from build123d import *

# Parameters (mm, degrees)
BOSS_EXTRUDE1_DEPTH      = 70
BOSS_EXTRUDE2_DEPTH      = 4
BOSS_EXTRUDE3_DEPTH      = 4
BOSS_EXTRUDE4_DEPTH      = 2
BOSS_EXTRUDE4_DEPTH_BACK = 2


with BuildPart() as part:
    # Sketch1 → Boss-Extrude1 (new body)
    with BuildSketch(Plane.XY):
        Polygon((0, 0), (30, 0), (30, 30), (26, 30), (26, 4), (0, 4), align=None)
    extrude(amount=BOSS_EXTRUDE1_DEPTH)

    # Sketch2 → Boss-Extrude2 (add)
    with BuildSketch(Plane.XY.offset(70)):
        Polygon((26, 30), (0, 4), (26, 4), align=None)
    extrude(amount=-BOSS_EXTRUDE2_DEPTH)

    # Sketch3 → Boss-Extrude3 (add)
    with BuildSketch(Plane(origin=(0, 0, 0), x_dir=(-1, 0, 0), z_dir=(0, 0, -1))):
        Polygon((-26, 30), (0, 4), (-26, 4), align=None)
    extrude(amount=-BOSS_EXTRUDE3_DEPTH)

    # Sketch4 → Boss-Extrude4 (add, two sides: drawn at the far end of the back side and taken through both)
    with BuildSketch(Plane(origin=(0, 0, 35), x_dir=(-1, 0, 0), z_dir=(0, 0, -1)).offset(-BOSS_EXTRUDE4_DEPTH_BACK)):
        Polygon((-26, 30), (-26, 4), (0, 4), align=None)
    extrude(amount=BOSS_EXTRUDE4_DEPTH + BOSS_EXTRUDE4_DEPTH_BACK)


solid = part.part
Input: part model. Units: mm. Frame: model coordinates. A direction names the side the tool comes from. Coordinates: 2 decimals unless noted, no trailing zeros. Order: outer loops, then holes, each group sorted by start corner. A loop starts at its lowest first (then second) coordinate and runs counter-clockwise, first axis right, second up.
1. Ray query, line 1 along Z through (x, y) = (7, 10); line 2 along X through (y, z) = (15.75, 53); line 3 along Y through (x, z) = (24, 58.5). Return the intervals inside material, ascending.
Checked values:
line 1: z = 0 to 4, 33 to 37, 66 to 70
line 2: x = 26 to 30
line 3: y = 0 to 4
2. Access query for faces 5 (the flat face through (13, 17, 68)), 6 (the flat face through (26, 17, 18)). Directions: +Z, -Z, +X, -X, +Y, -Y. A direction counts if a zero-diameter tool reaches every point of the face in a straight line with its end or side. Return the directions, or none.
Checked values:
face 5: +Z, -Z, -X, +Y
face 6: -X, +Y
3. Cut plane A-A, the plane x = 10.25. Return loops of the section in (y, z), plus the area to 3 significant figures.
Checked values:
outline: (0, 0) - (14.25, 0) - (14.25, 4) - (4, 4) - (4, 33) - (14.25, 33) - (14.25, 37) - (4, 37) - (4, 66) - (14.25, 66) - (14.25, 70) - (0, 70) - close
area: 403 mm2
4. Draft query along Z for faces 1 (the flat face through (18, 12, 0)), 2 (the flat face through (19, 11, 66)), 3 (the flat face through (18, 12, 70)), 4 (the flat face through (30, 15, 35)). Return one class per face: +Z half, -Z half, draft (parallel to the pull), parting line (faces both ways), or undercut.
Checked values:
face 1: -Z half
face 2: undercut
face 3: +Z half
face 4: draft
5. Cut plane B-B, the plane y = 12.25. Return loops of the section in (x, z), plus the area to 3 significant figures.
Checked values:
outline: (8.25, 0) - (30, 0) - (30, 70) - (8.25, 70) - (8.25, 66) - (26, 66) - (26, 37) - (8.25, 37) - (8.25, 33) - (26, 33) - (26, 4) - (8.25, 4) - close
area: 493 mm2
6. Contact query for flat-ended pins moving along their axis: P1, Ø1.5, axis at x = 22.5, z = 36.5, coming from the +Y side; P2, Ø1, axis at y = 27, z = 59.5, coming from the -X side; P3, Ø3, axis at x = 22.5, z = 12.5, coming from the -Y side; P4, Ø8, axis at x = 11.5, z = 45, coming from the +Y side. Output: stop coordinate, or through.
Checked values:
P1: stops at y = 27.25
P2: stops at x = 26
P3: stops at y = 0
P4: stops at y = 4
7. Cut plane C-C, the plane z = 36. Return loops of the section in (x, y), plus the area to 3 significant figures.
Checked values:
outline: (0, 0) - (30, 0) - (30, 30) - (26, 30) - (0, 4) - close
area: 562 mm2
8. Cut plane D-D, the plane z = 13. Return loops of the section in (x, y), plus the area to 3 significant figures.
Checked values:
outline: (0, 0) - (30, 0) - (30, 30) - (26, 30) - (26, 4) - (0, 4) - close
area: 224 mm2
